```python
from build123d import *

# Parameters (mm, degrees)
SWEEP1_START        = -19.69
SWEEP1_OUTLINE_R    = 2.5
SWEEP1_DEPTH        = 38.69
SWEEP1_START_2      = -12
SWEEP1_2_OUTLINE_R  = 2.5
SWEEP1_2_DEPTH      = 44.35
SWEEP1_3_OUTLINE_R  = 2.5
SWEEP1_3_ANGLE      = 90
DOME1_FACE_RADIUS   = 2.5
DOME1_HEIGHT        = 3
DOME2_FACE_RADIUS   = 2.5
DOME2_HEIGHT        = 3
EXTRUDE1_REACH      = 51.69
EXTRUDE1_END_RADIUS = 2.5
SKETCH3_W           = 33
SKETCH3_H           = 5


with BuildPart() as part:
    # Sweep1: read off the stored shape, not the designer's step
    # Sweep1 outline → Sweep1 (new body)
    with BuildSketch(Plane.YZ.offset(SWEEP1_START)):
        with Locations((4, 38.35)):
            Circle(SWEEP1_OUTLINE_R)
    extrude(amount=SWEEP1_DEPTH)



with BuildPart() as body_2:
    # Sweep1 2 outline → Sweep1 2 (new body)
    with BuildSketch(Plane.XY.offset(SWEEP1_START_2)):
        with Locations((25, 4)):
            Circle(SWEEP1_2_OUTLINE_R)
    extrude(amount=SWEEP1_2_DEPTH)


with BuildPart() as part_1:
    add(part.part)

    add(body_2.part)  # Sweep1 3 merges body 2
    # Sweep1 3 outline → Sweep1 3 (revolve)
    with BuildSketch(Plane(origin=(19, 0, 32.35), x_dir=(0, 0, 1), z_dir=(-1, 0, 0))):
        with Locations((6, 4)):
            Circle(SWEEP1_3_OUTLINE_R)
    revolve(axis=Axis((19, 0, 32.35), (0, 1, 0)), revolution_arc=SWEEP1_3_ANGLE)

    # Dome1: a dome of height H over a round flat face of radius A is a cap of a sphere of radius (A * A + H * H) / (2 * H)
    dome1_r = (DOME1_FACE_RADIUS * DOME1_FACE_RADIUS + DOME1_HEIGHT * DOME1_HEIGHT) / (2 * DOME1_HEIGHT)
    dome1_base = Plane((-19.69, 4, 38.35), z_dir=(-1, 0, 0))
    with Locations(dome1_base.offset(DOME1_HEIGHT - dome1_r)):
        dome1_ball = Sphere(dome1_r, mode=Mode.PRIVATE)
    add(split(dome1_ball, bisect_by=dome1_base, keep=Keep.TOP, mode=Mode.PRIVATE))

    # Dome2: a dome of height H over a round flat face of radius A is a cap of a sphere of radius (A * A + H * H) / (2 * H)
    dome2_r = (DOME2_FACE_RADIUS * DOME2_FACE_RADIUS + DOME2_HEIGHT * DOME2_HEIGHT) / (2 * DOME2_HEIGHT)
    dome2_base = Plane((25, 4, -12), z_dir=(0, 0, -1))
    with Locations(dome2_base.offset(DOME2_HEIGHT - dome2_r)):
        dome2_ball = Sphere(dome2_r, mode=Mode.PRIVATE)
    add(split(dome2_ball, bisect_by=dome2_base, keep=Keep.TOP, mode=Mode.PRIVATE))

    # Extrude1: up to this cylinder (the profile starts outside it)
    extrude1_end = Plane(origin=(-3.19, 4, 38.35), z_dir=(-1, 0, 0)) * Cylinder(EXTRUDE1_END_RADIUS, 109.38, mode=Mode.PRIVATE)
    # Sketch3 → Extrude1 (add, up to the surface)
    with BuildSketch(Plane(origin=(0, 0.34, 0), x_dir=(-1, 0, 0), z_dir=(0, 1, 0)), mode=Mode.PRIVATE) as extrude1_sk1:
        with Locations((3.19, 38.35)):
            Rectangle(SKETCH3_W, SKETCH3_H)
    extrude1_tool1 = extrude(extrude1_sk1.sketch, amount=EXTRUDE1_REACH, mode=Mode.PRIVATE) - extrude1_end
    add(extrude1_tool1.solids().sort_by_distance((-3.19, 0.34, 38.35))[0])


solid = part_1.part
```
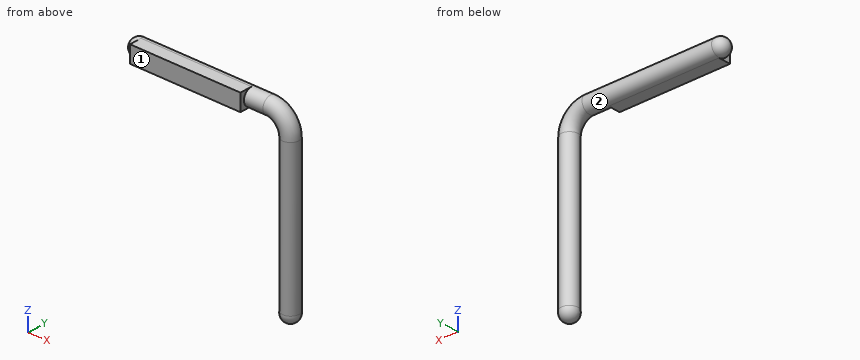
The listing builds one solid part. Answer for the finished solid, in the listing's coordinates (mm). Face numbers are marked on the shaded views. A direction names the side the tool comes from. Coordinates: 2 decimals unless noted, no trailing zeros. Loops run counter-clockwise (first coordinate to the right, second up) from the corner with the lowest first, then second, coordinate; pieces in that order, holes last. Notation, with made-up numbers: (6.5, -36) -> (53.5, -36) arc R4 cw to (53.5, -32) -> close; hole circle Ø2 at (-31.75, -28). An arc over 180 degrees is marked (long way). Return JSON: item names as keys, results as strings. Group by question number.
(1) Find the intervals of material crossed by probe 1 along Z at (x, y) = (-15, 2.25); probe 2 along X at (y, z) = (6, 19); probe 3 along Y at (x, z) = (25.5, -3.5), in increasing order. Write a range as from..to.
(2) Given pin 1 Ø1 at (x, y) = (13, 4.5) entering from +Z; pin 2 Ø1.1 at (y, z) = (1.5, 39.5) entering from -X; pin 3 Ø3 at (x, y) = (-6.5, 2.5) entering from -Z, each flat-ended and moving along its own axis, determine where each tip first touches the part or whether it passes through.
(3) Which of the six approach directions +Z, -Z, +X, -X, +Y, -Y give full straight-line access (tool end or side, diameter ignored) to the marked faces 1 and 2?
(4) A cutting plane is placed at C-C on x = 5.5. Write down the section's boundary in (y, z).
(5) A cutting plane is placed at A-A on y = 5.5. Write down the section's boundary in (x, z).
(6) A cutting plane is placed at B-B on z = 4. Write down the section's boundary in (x, y), and give its area (3 significant figures).
The answers:
{
 "1": {"probe 1": "z = 35.85..40.85", "probe 2": "x = 23.5..26.5", "probe 3": "y = 1.55..6.45"},
 "2": {"pin 1": "stops at z = 40.85", "pin 2": "stops at x = -21.42", "pin 3": "stops at z = 35.85"},
 "3": {"face 1": "+Z, -Z, +X, -X, -Y", "face 2": "none"},
 "4": {"outline": "(0.34, 35.85) -> (4, 35.85) arc R2.5 ccw to (4, 40.85) -> (0.34, 40.85) -> close"},
 "5": {"outline": "(-19.69, 36.35) -> (19, 36.35) arc R4 cw to (23, 32.35) -> (23, -12) arc R2.05 ccw (long way) to (27, -12) -> (27, 32.35) arc R8 ccw to (19, 40.35) -> (-19.69, 40.35) arc R2.05 ccw (long way) to start"},
 "6": {"outline": "circle Ø5 at (25, 4)", "area": "19.6 mm^2"}
}
